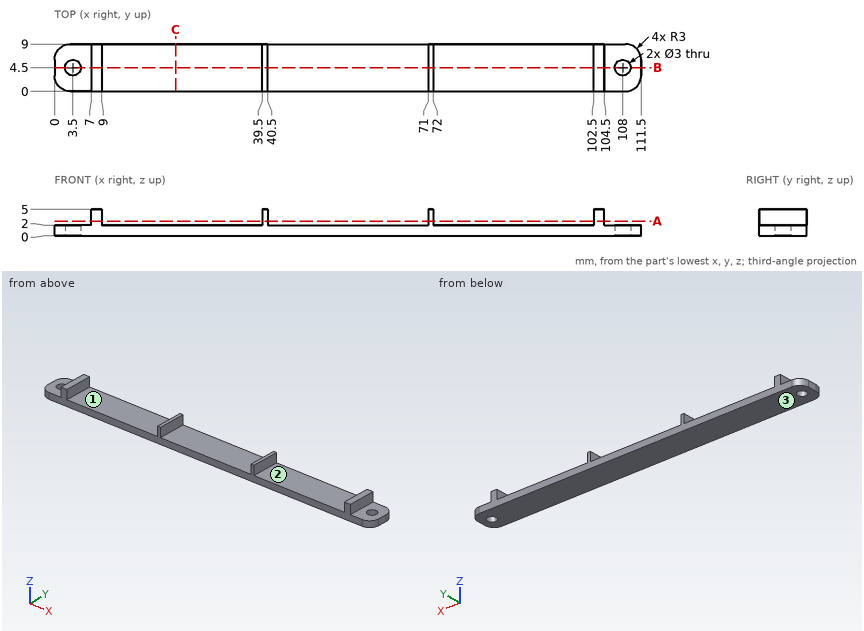
Verification items for this drawing (mm, ordinates from the low corner). Round coordinates to 2 decimals unless told otherwise and drop trailing zeros. Order: outer loops, then holes, each group sorted by start corner. A loop starts at its lowest first (then second) coordinate and runs counter-clockwise, first axis right, second up. Notation, with made-up numbers: (51.25, -31.5) - (63.25, -31.5) arc R22 cw to (63.25, 6.5) - close; hole circle Ø7 at (31.25, 63). An arc over 180 degrees is marked (long way). Use CSV: the item, a comma, the result in double quotes. Start each with the question number.
1) Mould release check, pull along X, two halves, no side actions. Record for the marked faces 1, 2 and 3: +X half, -X half, draft (parallel to the pull), parting line (faces both ways), or undercut.
2) Section check C-C, the plane x = 23. Record the cut outline in (y, z).
3) Thickness scan on L1, parallel to X at y = 4.5, z = 1.15; L2, parallel to X at y = 7.25, z = 2.25; L3, parallel to Y at x = 3.5, z = 0.65. Record the ranges inside material, lowest first.
4) Go/stop test with flat-tipped pins: P1, Ø1.5, axis at y = 6.5, z = 4, coming from the +X side; P2, Ø2.5, axis at y = 5.5, z = 4, coming from the -X side; P3, Ø1.5, axis at y = 1, z = 2, coming from the +X side. Record where each tip stops, or that it passes through.
5) Section check A-A, the plane z = 2.75. Record the cut outline in (x, y), plus the area to 3 significant figures.
6) Section check B-B, the plane y = 4.5. Record the cut outline in (x, z), plus the area to 3 significant figures.
Answers:
1,face 1,"undercut"
1,face 2,"undercut"
1,face 3,"draft"
2,outline,"(0, 0) - (9, 0) - (9, 2) - (0, 2) - close"
3,L1,"x = 0 to 2, 5 to 106.5, 109.5 to 111.5"
3,L2,"x = 7 to 9, 39.5 to 40.5, 71 to 72, 102.5 to 104.5"
3,L3,"y = 0 to 3, 6 to 9"
4,P1,"stops at x = 104.5"
4,P2,"stops at x = 7"
4,P3,"stops at x = 111.23"
5,outline,"(7, 0) - (9, 0) - (9, 9) - (7, 9) - close; (39.5, 0) - (40.5, 0) - (40.5, 9) - (39.5, 9) - close; (71, 0) - (72, 0) - (72, 9) - (71, 9) - close; (102.5, 0) - (104.5, 0) - (104.5, 9) - (102.5, 9) - close"
5,area,"54.0 mm²"
6,outline,"(0, 0) - (2, 0) - (2, 2) - (0, 2) - close; (5, 0) - (106.5, 0) - (106.5, 2) - (104.5, 2) - (104.5, 5) - (102.5, 5) - (102.5, 2) - (72, 2) - (72, 5) - (71, 5) - (71, 2) - (40.5, 2) - (40.5, 5) - (39.5, 5) - (39.5, 2) - (9, 2) - (9, 5) - (7, 5) - (7, 2) - (5, 2) - close; (109.5, 0) - (111.5, 0) - (111.5, 2) - (109.5, 2) - close"
6,area,"229 mm²"
